Could you check a few things on this drawing? It's one solid part, dimensions in mm from its lowest x, y, z. Give positions to 0.01 mm unless a question says otherwise; leave off trailing zeros. Order: outer loops, then holes, each group sorted by start corner. A loop starts at its lowest first (then second) coordinate and runs counter-clockwise, first axis right, second up. Notation, with made-up numbers: M -22.5,63.25 L 34.5,63.25 A21 cw 34.5,91.25 Z; hole C -35.75,51.25 d10. An arc over 180 degrees is marked long. Use one line per item in the form item = value. Start each with the question number.
1. I want a section at A-A, the plane x = 4.9. List the corners of the cut face in (y, z) for me.
2. I want a section at B-B, the plane y = 1.7. List the corners of the cut face in (x, z) for me, and give its area (3 significant figures).
3. I want a section at C-C, the plane z = 24.75. List the corners of the cut face in (x, y) for me.
4. I need wall thicknesses on L1, parallel to Z at x = 0.8, y = 1.1; L2, parallel to X at y = 3.15, z = 20.5. Which ranges of each line are inside material? Lowest first, please.
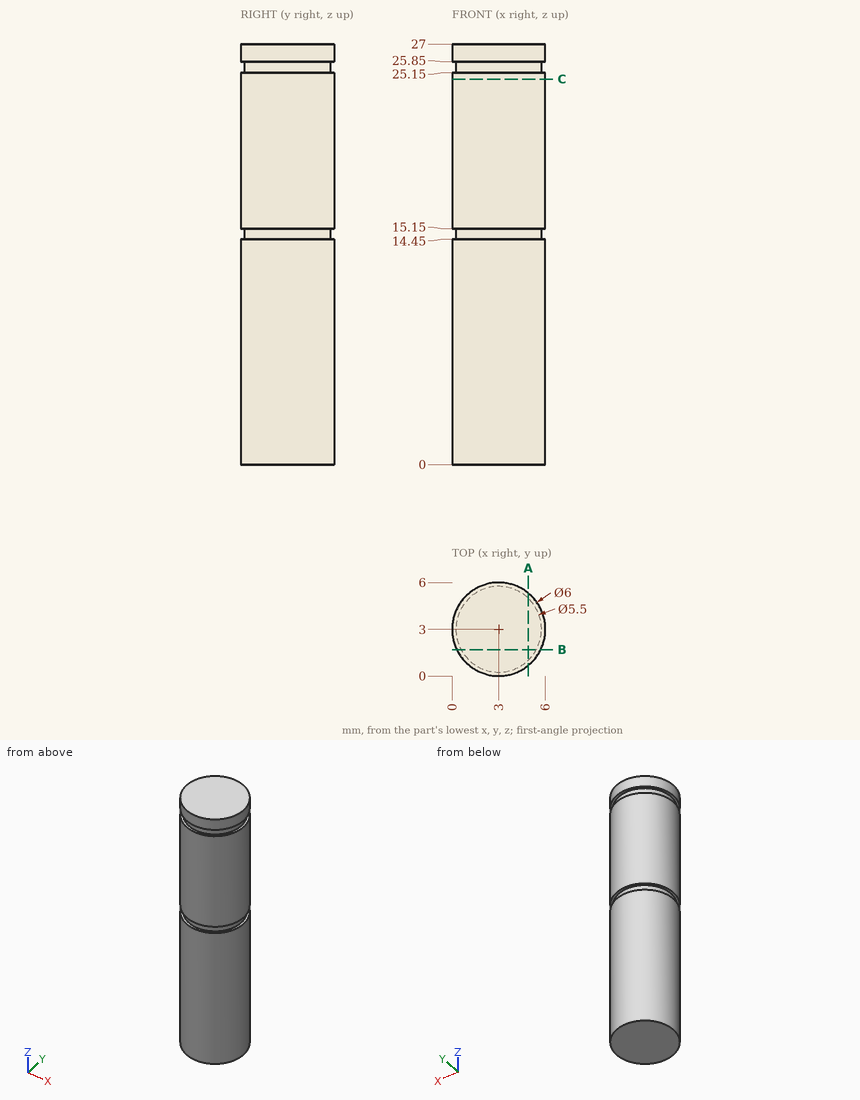
Check result:
q1.outline = M 0.68,0 L 5.32,0 L 5.32,14.45 L 4.99,14.45 L 4.99,15.15 L 5.32,15.15 L 5.32,25.15 L 4.99,25.15 L 4.99,25.85 L 5.32,25.85 L 5.32,27 L 0.68,27 L 0.68,25.85 L 1.01,25.85 L 1.01,25.15 L 0.68,25.15 L 0.68,15.15 L 1.01,15.15 L 1.01,14.45 L 0.68,14.45 Z
q2.outline = M 0.3,0 L 5.7,0 L 5.7,14.45 L 5.42,14.45 L 5.42,15.15 L 5.7,15.15 L 5.7,25.15 L 5.42,25.15 L 5.42,25.85 L 5.7,25.85 L 5.7,27 L 0.3,27 L 0.3,25.85 L 0.58,25.85 L 0.58,25.15 L 0.3,25.15 L 0.3,15.15 L 0.58,15.15 L 0.58,14.45 L 0.3,14.45 Z
q2.area = 145 mm2
q3.outline = C 3,3 d6
q4.L1 = 0 to 14.45, 15.15 to 25.15, 25.85 to 27
q4.L2 = 0 to 6
